Design review of the part built by this model. Coordinates are the model's own, in mm. A direction names the side the tool comes from. Coordinates: 2 decimals unless noted, no trailing zeros. Loops run counter-clockwise (first coordinate to the right, second up) from the corner with the lowest first, then second, coordinate; pieces in that order, holes last. Notation, with made-up numbers: (52, 37.25) - (107, 37.25) arc R15 cw to (107, 63.25) - close; hole circle Ø2 at (66.5, -23). An arc over 180 degrees is marked (long way). Answer in a Markdown table with one row per item. Add a question column.
(1) To check wall thickness, follow L1, parallel to Z at x = -80.5, y = -56.5; L2, parallel to Z at x = -19.5, y = -132; L3, parallel to Y at x = -7.5, z = -45.5. State the ranges of each line that lie inside material, in increasing order. Write a range as [from, to].
(2) Clearance check with flat-ended pins moving along their axes: pin 1 (24 mm diameter, centred on x = -145.5, z = -24, fed in from +Y); pin 2 (10 mm diameter, centred on y = -87.5, z = -58, fed in from -X); pin 3 (21.5 mm diameter, centred on x = -50, z = 93, fed in from -Y); pin 4 (22 mm diameter, centred on y = -107.5, z = 31.5, fed in from -X). State where each tip first meets the part, or that it passes through.
(3) We need section C-C, the plane z = -51.5. Write out the cut boundary in (x, y).
(4) We need section B-B, the plane y = 13.5. Write out the cut boundary in (x, z), plus the area to 3 significant figures.
(5) We need section A-A, the plane x = 41. Write out the cut boundary in (y, z).
(6) For faces 1 (the face through (-69, -157.96, -98)), 2 (the face through (-69, -157.96, 94)), 3 (the face through (-149.546, -116, 2)), 4 (the face through (1.5, -135.05, 1.55)), 5 (the face through (-51.7, -67.1, 1.2)), list the 3-axis set-ups (+Z, -Z, +X, -X, +Y, -Y) from which the entire face can be reached by the end or side of a thin tool; tool diameter is ignored.
(7) We need section D-D, the plane z = 0. Write out the cut boundary in (x, y).
from build123d import *

# Parameters (mm, degrees)
BOSS_EXTRUDE1_DEPTH      = 110.5
BOSS_EXTRUDE1_DEPTH_BACK = 110.5
CUT_EXTRUDE1_DEPTH       = 85.5
CUT_EXTRUDE1_DEPTH_BACK  = 85.5
SKETCH3_R                = 90
BOSS_EXTRUDE2_DEPTH      = 20
BODY_MOVE_COPY1_ANGLE    = 90
BOSS_EXTRUDE3_DEPTH      = 1


with BuildPart() as part:
    # Sketch1 → Boss-Extrude1 (new, two sides: drawn at the far end of the back side and taken through both)
    with BuildSketch(Plane(origin=(0, 0, 0), x_dir=(0, 0, -1), z_dir=(1, 0, 0)).offset(-BOSS_EXTRUDE1_DEPTH_BACK)):
        with BuildLine():
            Line((-64.292863754, -51.10932545), (55.707136246, -51.10932545))
            ThreePointArc((55.707136246, -51.10932545), (69.84927187, -45.251461074), (75.707136246, -31.10932545))
            Line((75.707136246, -31.10932545), (75.707136246, 12.89067455))
            Line((75.707136246, 12.89067455), (-26.557571018, 143.789344322))
            ThreePointArc((-26.557571018, 143.789344322), (-105.517875867, 157.806043193), (-127.885671837, 80.793840961))
            Line((-127.885671837, 80.793840961), (-64.292863754, -51.10932545))
        make_face()
    extrude(amount=BOSS_EXTRUDE1_DEPTH + BOSS_EXTRUDE1_DEPTH_BACK)

    # Sketch2 → Cut-Extrude1 (cut, two sides: drawn at the far end of the back side and taken through both)
    with BuildSketch(Plane(origin=(0, 0, 0), x_dir=(0, 0, -1), z_dir=(1, 0, 0)).offset(-CUT_EXTRUDE1_DEPTH_BACK)):
        with BuildLine():
            Line((-127.885671837, 80.793840961), (-81.149808611, -16.144925076))
            ThreePointArc((-81.149808611, -16.144925076), (-21.055510127, 40.123069763), (60.857619094, 31.898033921))
            Line((60.857619094, 31.898033921), (-26.557571018, 143.789344322))
            ThreePointArc((-26.557571018, 143.789344322), (-105.517875867, 157.806043193), (-127.885671837, 80.793840961))
        make_face()
    extrude(amount=CUT_EXTRUDE1_DEPTH + CUT_EXTRUDE1_DEPTH_BACK, mode=Mode.SUBTRACT)

    # Sketch3 → Boss-Extrude2 (add)
    with BuildSketch(Plane.XZ.offset(51.10932545)):
        with Locations(Location((0, 4.292863754, 0), (0, 0, 41.810314896))):
            Circle(SKETCH3_R)
    extrude(amount=BOSS_EXTRUDE2_DEPTH)


with BuildPart() as part_1:
    # Body-Move_Copy1: moved
    add(part.part.rotate(Axis((0, 0, 0), (0, 1, 0)), BODY_MOVE_COPY1_ANGLE))

    # Sketch4 → Boss-Extrude3 (add)
    with BuildSketch(Plane.XY.offset(110.5)):
        with BuildLine():
            add(Edge.make_bspline(
                [(-7.892298412, 36.986704623), (-7.731424988, 36.97864928), (-7.419070809, 36.963008908), (-6.967618916, 36.851284273), (-6.555873051, 36.656661621), (-6.188786467, 36.392582396), (-5.87896222, 36.078180341), (-5.65016273, 35.71921506), (-5.513989502, 35.321796415), (-5.497073858, 35.044635312), (-5.488452259, 34.90337129)],
                knots=[0, 0, 0, 0, 1.093025379, 2.122233962, 3.13739964, 4.170167025, 5.181202767, 6.119320369, 7.041451468, 8, 8, 8, 8], degree=3))
            add(Edge.make_bspline(
                [(-5.488452259, 34.90337129), (-5.497406625, 34.765509384), (-5.515182791, 34.491826572), (-5.649926135, 34.097337276), (-5.880505469, 33.738380755), (-6.18693796, 33.41913881), (-6.555993835, 33.154861618), (-6.968359777, 32.961898769), (-7.418241254, 32.842085164), (-7.731283731, 32.827526345), (-7.892298412, 32.820037956)],
                knots=[0, 0, 0, 0, 0.937343707, 1.860810353, 2.800286657, 3.820978539, 4.855241709, 5.871877678, 6.905391563, 8, 8, 8, 8], degree=3))
            add(Edge.make_bspline(
                [(-7.892298412, 32.820037956), (-8.053339268, 32.827461421), (-8.366432635, 32.841894016), (-8.817422774, 32.963004322), (-9.232383344, 33.153609982), (-9.602694964, 33.417641247), (-9.90389839, 33.740107583), (-10.134877578, 34.097146255), (-10.26936178, 34.491874817), (-10.287172696, 34.765525545), (-10.296144566, 34.90337129)],
                knots=[0, 0, 0, 0, 1.094267983, 2.127460414, 3.154075327, 4.188016812, 5.200584313, 6.139768412, 7.062947834, 8, 8, 8, 8], degree=3))
            add(Edge.make_bspline(
                [(-10.296144566, 34.90337129), (-10.287504989, 35.044618426), (-10.27055407, 35.321746398), (-10.134639162, 35.71940767), (-9.905453118, 36.07643862), (-9.600833421, 36.394095039), (-9.23250791, 36.657911588), (-8.818168555, 36.850199857), (-8.365603653, 36.963201799), (-8.053198229, 36.978714853), (-7.892298412, 36.986704623)],
                knots=[0, 0, 0, 0, 0.95825844, 1.880110469, 2.817944164, 3.820814674, 4.853269506, 5.878408302, 6.90730541, 8, 8, 8, 8], degree=3))
        make_face()
    extrude(amount=BOSS_EXTRUDE3_DEPTH)


with BuildPart() as part_2:
    # Body-Move_Copy2: moved
    add(part_1.part.moved(Location((-73.839012149, -106.85067455, 0))))


solid = part_2.part
Responses:
| question | item | result |
|---|---|---|
| 1 | L1 | z = [-110.5, -85.5], [85.5, 110.5] |
| 1 | L2 | z = [-110.5, 110.5] |
| 1 | L3 | y = [-177.96, -157.96], [-153.72, -98.16] |
| 2 | pin 1 | stops at y = -74.27 |
| 2 | pin 2 | stops at x = -148.41 |
| 2 | pin 3 | stops at y = -177.96 |
| 2 | pin 4 | stops at x = -149.55 |
| 3 | outline | (-149.55, -137.96) arc R20 ccw to (-129.55, -157.96) - (-143.36, -157.96) - (-143.36, -177.96) - (4.26, -177.96) - (4.26, -157.96) - (-9.55, -157.96) - (7.31, -123) arc R99.55 ccw to (-134.7, -74.95) - (-149.55, -93.96) - close |
| 4 | outline | (-65.59, -110.5) - (58.46, -110.5) - (58.46, -85.5) - (-65.59, -85.5) - close; (-65.59, 85.5) - (58.46, 85.5) - (58.46, 110.5) - (-65.59, 110.5) - close |
| 4 | area | 6,200 mm2 |
| 5 | outline | (-53.12, -110.5) - (43.81, -110.5) - (43.81, -85.5) - (-53.12, -85.5) - close; (-53.12, 85.5) - (43.81, 85.5) - (43.81, 110.5) - (-53.12, 110.5) - close |
| 6 | face 1 | -Z, -Y |
| 6 | face 2 | +Z, -Y |
| 6 | face 3 | +Z, -Z, -X, +Y |
| 6 | face 4 | +Z, -Z, +X |
| 6 | face 5 | +Y |
| 7 | outline | (-159.55, -177.96) - (20.45, -177.96) - (20.45, -157.96) - (-9.55, -157.96) - (7.31, -123) arc R99.55 ccw to (-134.7, -74.95) - (-149.55, -93.96) - (-149.55, -137.96) arc R20 ccw to (-129.55, -157.96) - (-159.55, -157.96) - close |
